Here's how the part is built. I have some questions about the finished solid (model axes, mm). Face numbers are marked on the shaded views. A direction names the side the tool comes from. Give positions to 0.01 mm unless a question says otherwise; leave off trailing zeros. Order: outer loops, then holes, each group sorted by start corner. A loop starts at its lowest first (then second) coordinate and runs counter-clockwise, first axis right, second up. Notation, with made-up numbers: M 34.25,83.25 L 74.25,83.25 A17 ccw 74.25,116.25 Z; hole C 7,15.25 d10. An arc over 180 degrees is marked long. Use CSV: the item, a comma, the result in double quotes. Start each with the question number.
```python
from build123d import *

# Parameters (mm, degrees)
EXTRUDE_START   = 2.5
SKETCH_1_W      = 24
SKETCH_1_H      = 10
SKETCH_1_R      = 1.5
EXTRUDE_1_DEPTH = 3
EXTRUDE_START_2 = -2.5
SKETCH_2_W      = 24
SKETCH_2_H      = 10
SKETCH_2_R      = 1.5
EXTRUDE_2_DEPTH = 3
SKETCH_3_W      = 24
SKETCH_3_H      = 11
EXTRUDE_3_DEPTH = 3
SKETCH_4_W      = 24
SKETCH_4_H      = 3
EXTRUDE_4_DEPTH = 16
EXTRUDE_5_DEPTH = 24
FILLET_1_R      = 0.2
FILLET_2_R      = 2


with BuildPart() as part:
    # Sketch 1 → Extrude 1 (new body)
    with BuildSketch(Plane.XY.offset(EXTRUDE_START)):
        Rectangle(SKETCH_1_W, SKETCH_1_H)
        with Locations((-7, 1)):
            Circle(SKETCH_1_R, mode=Mode.SUBTRACT)
        with Locations(Location((7, 1, 0), (0, 0, 180))):
            Circle(SKETCH_1_R, mode=Mode.SUBTRACT)
    extrude(amount=EXTRUDE_1_DEPTH)



with BuildPart() as body_2:
    # Sketch 2 → Extrude 2 (new body)
    with BuildSketch(Plane.XY.offset(EXTRUDE_START_2)):
        Rectangle(SKETCH_2_W, SKETCH_2_H)
        with Locations(Location((7, 1, 0), (0, 0, 180))):
            Circle(SKETCH_2_R, mode=Mode.SUBTRACT)
        with Locations((-7, 1)):
            Circle(SKETCH_2_R, mode=Mode.SUBTRACT)
    extrude(amount=-EXTRUDE_2_DEPTH)


with BuildPart() as part_1:
    add(part.part)

    add(body_2.part)  # Extrude 3 merges body 2
    # Sketch 3 → Extrude 3 (add)
    with BuildSketch(Plane(origin=(0, 5, 0), x_dir=(1, 0, 0), z_dir=(0, 1, 0))):
        Rectangle(SKETCH_3_W, SKETCH_3_H)
    extrude(amount=EXTRUDE_3_DEPTH)

    # Sketch 4 → Extrude 4 (add)
    with BuildSketch(Plane.XY.offset(5.5)):
        with Locations((0, 6.5)):
            Rectangle(SKETCH_4_W, SKETCH_4_H)
    extrude(amount=EXTRUDE_4_DEPTH)

    # Sketch 5 → Extrude 5 (add)
    with BuildSketch(Plane(origin=(12, 0, 0), x_dir=(0, 0, -1), z_dir=(1, 0, 0))):
        Polygon((-18.5, 5), (-17.3, 3.5), (-19.7, 3.5), align=None)
        Polygon((-18.9, 4.5), (-18.5, 5), (-18.9, 5), align=None)
        Polygon((-18.1, 5), (-18.5, 5), (-18.1, 4.5), align=None)
    extrude(amount=-EXTRUDE_5_DEPTH)

    # Fillet 1
    fillet_1_edges = [part_1.edges().sort_by_distance(p)[0] for p in [
        (0, 3.5, 17.3),
        (0, 3.5, 19.7),
    ]]
    fillet(fillet_1_edges, radius=FILLET_1_R)

    # Fillet 2
    fillet_2_edges = [part_1.edges().sort_by_distance(p)[0] for p in [
        (-12, 8, 8),
        (12, 8, 8),
    ]]
    fillet(fillet_2_edges, radius=FILLET_2_R)


solid = part_1.part
```
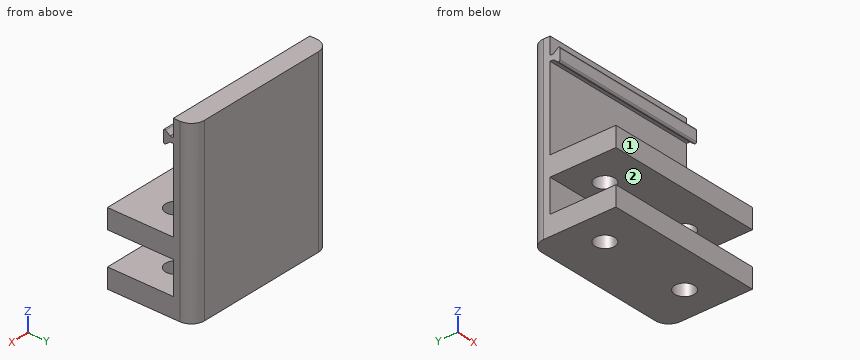
Q1. For P1, Ø0.8, axis at x = 4, z = 19, coming from the -Y side; P2, Ø4, axis at x = -4.5, z = 9, coming from the -Y side, each with a flat end and sliding along its axis, tell me the tip position at first contact or that it passes through.
Q2. Imagine slicing it at A-A, the plane z = 4. Please give me the cut outline in (x, y), then the cut area to 3 significant figures.
Q3. Imagine slicing it at C-C, the plane y = 1. Please give me the cut outline in (x, z), then the cut area to 3 significant figures.
Q4. Imagine slicing it at D-D, the plane x = 3. Please give me the cut outline in (y, z).
Q5. Imagine slicing it at B-B, the plane x = -7. Please give me the cut outline in (y, z).
Q6. For the marked faces 1 and 2, which set-ups out of +Z, -Z, +X, -X, +Y, -Y let a thin tool reach every point of the face, with its end or its side?
Q7. I need wall thicknesses on line 1 (Z direction, x = -8, y = 4.5); line 2 (Z direction, x = 10.25, y = -0.25); line 3 (Z direction, x = 8.5, y = 4.25). Which ranges of each line are inside material? Lowest first, please. Write a range as [from, to].
Reply:
1,P1,"stops at y = 3.5"
1,P2,"stops at y = 5"
2,outline,"M -12,-5 L 12,-5 L 12,6 A2 ccw 10,8 L -10,8 A2 ccw -12,6 Z; hole C -7,1 d3; hole C 7,1 d3"
2,area,"296 mm^2"
3,outline,"M -12,-5.5 L -8.5,-5.5 L -8.5,-2.5 L -12,-2.5 Z; M -12,2.5 L -8.5,2.5 L -8.5,5.5 L -12,5.5 Z; M -5.5,-5.5 L 5.5,-5.5 L 5.5,-2.5 L -5.5,-2.5 Z; M -5.5,2.5 L 5.5,2.5 L 5.5,5.5 L -5.5,5.5 Z; M 8.5,-5.5 L 12,-5.5 L 12,-2.5 L 8.5,-2.5 Z; M 8.5,2.5 L 12,2.5 L 12,5.5 L 8.5,5.5 Z"
3,area,"108 mm^2"
4,outline,"M -5,-5.5 L 8,-5.5 L 8,21.5 L 5,21.5 L 5,18.9 L 4.5,18.9 L 3.82,19.44 A0.2 ccw 3.5,19.28 L 3.5,17.72 A0.2 ccw 3.82,17.56 L 4.5,18.1 L 5,18.1 L 5,5.5 L -5,5.5 L -5,2.5 L 5,2.5 L 5,-2.5 L -5,-2.5 Z"
5,outline,"M -5,-5.5 L -0.5,-5.5 L -0.5,-2.5 L -5,-2.5 Z; M -5,2.5 L -0.5,2.5 L -0.5,5.5 L -5,5.5 Z; M 2.5,-5.5 L 8,-5.5 L 8,21.5 L 5,21.5 L 5,18.9 L 4.5,18.9 L 3.82,19.44 A0.2 ccw 3.5,19.28 L 3.5,17.72 A0.2 ccw 3.82,17.56 L 4.5,18.1 L 5,18.1 L 5,5.5 L 2.5,5.5 L 2.5,2.5 L 5,2.5 L 5,-2.5 L 2.5,-2.5 Z"
6,face 1,"+Z, -Z, +X, -X, -Y"
6,face 2,"+X, -X, -Y"
7,line 1,"z = [-5.5, -2.5], [2.5, 5.5], [18.1, 18.9]"
7,line 2,"z = [-5.5, -2.5], [2.5, 5.5]"
7,line 3,"z = [-5.5, -2.5], [2.5, 5.5], [17.9, 19.1]"
